Build history of the part. All positions in model axes, mm. Give positions to 0.01 mm unless a question says otherwise; leave off trailing zeros. Order: outer loops, then holes, each group sorted by start corner. A loop starts at its lowest first (then second) coordinate and runs counter-clockwise, first axis right, second up. Notation, with made-up numbers: (51, 43.5) -> (78, 43.5) arc R23 ccw to (78, 79.5) -> close; hole circle Ø1 at (11.25, 83). An arc over 180 degrees is marked (long way). One line per question, with ' | ' between items. Start each with the question number.
(1) Cut at B-B (y = 0). Give the cut face in (x, z), then the cut area to 3 significant figures.
(2) Cut at A-A (x = 0). Give the cut face in (y, z).
(3) Cut at C-C (z = 3.5). Give the cut face in (x, y), then the cut area to 3 significant figures.
(4) Cut at D-D (y = 58). Give the cut face in (x, z), then the cut area to 3 significant figures.
(5) Pin check, flat tips, straight feed: pin 1 Ø4 at (y, z) = (26.5, 3) entering from -X; pin 2 Ø6 at (x, z) = (57.5, -2) entering from -Y; pin 3 Ø2 at (x, z) = (-20, 3) entering from +Y. Stop position of each tip, or through.
(6) Pull direction Y, two halves, no side cores. Call faces 1 (the face through (-1, -32, 5)), 2 (the face through (-9.764, 74.362, 0.07)), 3 (the face through (3.38, 60.15, 0.07)): +Y half, -Y half, draft (parallel to the pull), parting line (faces both ways), or undercut.
(7) Drill centre lines: L1, parallel to Y at x = 0, z = 0.75; L2, parallel to X at y = 1.5, z = 1.5 (3 decimals); L3, parallel to Y at x = -12, z = -1. Where is each one in solid material? Low to high. Write a range as from..to.
Solid Edge part; units mm, degrees
sketch "Sketch1" plane through (0, 0, 0) normal (0, 0, 1) x (1, 0, 0)
  circle A0 centre (0, 0) radius 75
  circle A1 centre (0, 0) radius 30
extrude "Protrusion1" add sketch "Sketch1" along normal mid plane 10
hole "Hole_1" at (0, 56.4641, 5) direction (0, 0, -1) diameter 10 end up to next
Result set:
1) outline: (-75, -5) -> (-30, -5) -> (-30, 5) -> (-75, 5) -> close; (30, -5) -> (75, -5) -> (75, 5) -> (30, 5) -> close | area: 900 mm2
2) outline: (-75, -5) -> (-30, -5) -> (-30, 5) -> (-75, 5) -> close; (30, -5) -> (51.46, -5) -> (51.46, 5) -> (30, 5) -> close; (61.46, -5) -> (75, -5) -> (75, 5) -> (61.46, 5) -> close
3) outline: circle Ø150 at (0, 0); hole circle Ø60 at (0, 0); hole circle Ø10 at (0, 56.46) | area: 14,800 mm2
4) outline: (-47.55, -5) -> (-4.76, -5) -> (-4.76, 5) -> (-47.55, 5) -> close; (4.76, -5) -> (47.55, -5) -> (47.55, 5) -> (4.76, 5) -> close | area: 856 mm2
5) pin 1: stops at x = -70.89 | pin 2: stops at y = -51.52 | pin 3: stops at y = 72.55
6) face 1: draft | face 2: parting line | face 3: undercut
7) L1: y = -75..-30, 30..51.46, 61.46..75 | L2: x = -74.985..-29.962, 29.962..74.985 | L3: y = -74.03..-27.5, 27.5..74.03
